```python
from build123d import *

# Parameters (mm, degrees)
CROQUIS1_W              = 800
CROQUIS1_H              = 342
SALIENTE_EXTRUIR1_DEPTH = 483
CROQUIS2_W              = 710
CROQUIS2_H              = 53.5
CORTAR_EXTRUIR1_DEPTH   = 483
CORTAR_EXTRUIR2_DEPTH   = 342
CORTAR_EXTRUIR4_DEPTH   = 800
VACIADO2_START          = -265.15812527
VACIADO2_OUTLINE_W      = 105
VACIADO2_OUTLINE_H      = 225
VACIADO2_DEPTH          = 530.31625054
VACIADO2_START_2        = -395
VACIADO2_2_DEPTH        = 790
VACIADO2_3_DEPTH        = 40
VACIADO2_START_3        = 355
VACIADO2_4_DEPTH        = 40
VACIADO2_START_4        = -112.5
VACIADO2_5_DEPTH        = 225
CROQUIS8_W              = 171
CROQUIS8_H              = 72.679369328
CORTAR_EXTRUIR7_DEPTH   = 113
CROQUIS9_W              = 171
CROQUIS9_H              = 72.679369328
CORTAR_EXTRUIR8_DEPTH   = 113


with BuildPart() as part:
    # Croquis1 → Saliente-Extruir1 (new body)
    with BuildSketch(Plane(origin=(0, 0, 0), x_dir=(1, 0, 0), z_dir=(0, 1, 0))):
        Rectangle(CROQUIS1_W, CROQUIS1_H)
    extrude(amount=SALIENTE_EXTRUIR1_DEPTH)

    # Croquis2 → Cortar-Extruir1 (cut)
    with BuildSketch(Plane(origin=(0, 483, 0), x_dir=(1, 0, 0), z_dir=(0, 1, 0))):
        with Locations((0, 144.25)):
            Rectangle(CROQUIS2_W, CROQUIS2_H)
        with Locations((0, -144.25)):
            Rectangle(CROQUIS2_W, CROQUIS2_H)
    extrude(amount=-CORTAR_EXTRUIR1_DEPTH, mode=Mode.SUBTRACT)

    # Croquis3 → Cortar-Extruir2 (cut)
    with BuildSketch(Plane.XY.offset(171)):
        Polygon((-355, 317.779645743), (-355, 0), (355, 0), (355, 317.779645743), (331.5, 317.779645743), (244, 422.779645743), (-244, 422.779645743), (-331.5, 317.779645743), align=None)
        Polygon((267.5, 483), (355, 378), (400, 378), (400, 483), align=None)
        Polygon((-400, 483), (-400, 378), (-355, 378), (-267.5, 483), align=None)
    extrude(amount=-CORTAR_EXTRUIR2_DEPTH, mode=Mode.SUBTRACT)

    # Croquis4 → Cortar-Extruir4 (cut)
    with BuildSketch(Plane(origin=(400, 0, 0), x_dir=(0, 0, -1), z_dir=(1, 0, 0))):
        Polygon((171, 378), (171, 70), (117.5, 378), align=None)
        Polygon((-171, 70), (-117.5, 378), (-171, 378), align=None)
        Polygon((-127.5, 45), (127.5, 45), (127.5, 75), (80, 325), (-80, 325), (-127.5, 75), align=None)
    extrude(amount=-CORTAR_EXTRUIR4_DEPTH, mode=Mode.SUBTRACT)

    # Vaciado2: read off the stored shape, not the designer's step
    # Vaciado2 outline → Vaciado2 (cut)
    with BuildSketch(Plane.YZ.offset(VACIADO2_START)):
        with Locations((425.5, 0)):
            Rectangle(VACIADO2_OUTLINE_W, VACIADO2_OUTLINE_H)
    extrude(amount=VACIADO2_DEPTH, mode=Mode.SUBTRACT)

    # Vaciado2 2 outline → Vaciado2 2 (cut)
    with BuildSketch(Plane.YZ.offset(VACIADO2_START_2)):
        Polygon((373, -112.5), (373, 112.5), (317.779645743, 112.5), (317.779645743, 81.371867309), (325, 80), (325, -80), (317.779645743, -81.371867309), (317.779645743, -112.5), align=None)
    extrude(amount=VACIADO2_2_DEPTH, mode=Mode.SUBTRACT)

    # Vaciado2 3 outline → Vaciado2 3 (cut)
    with BuildSketch(Plane.YZ.offset(VACIADO2_START_2)):
        Polygon((69.568973838, 166), (5, 166), (5, -166), (69.568973838, -166), (373, -113.293636689), (373, -112.5), (317.779645743, -112.5), (317.779645743, -81.371867309), (75, -127.5), (45, -127.5), (45, 127.5), (75, 127.5), (317.779645743, 81.371867309), (317.779645743, 112.5), (373, 112.5), (373, 113.293636689), align=None)
    extrude(amount=VACIADO2_3_DEPTH, mode=Mode.SUBTRACT)

    # Vaciado2 4 outline → Vaciado2 4 (cut)
    with BuildSketch(Plane.YZ.offset(VACIADO2_START_3)):
        Polygon((69.568973838, 166), (5, 166), (5, -166), (69.568973838, -166), (373, -113.293636689), (373, -112.5), (317.779645743, -112.5), (317.779645743, -81.371867309), (75, -127.5), (45, -127.5), (45, 127.5), (75, 127.5), (317.779645743, 81.371867309), (317.779645743, 112.5), (373, 112.5), (373, 113.293636689), align=None)
    extrude(amount=VACIADO2_4_DEPTH, mode=Mode.SUBTRACT)

    # Vaciado2 5 outline → Vaciado2 5 (cut)
    with BuildSketch(Plane.XY.offset(VACIADO2_START_4)):
        Polygon((352.65812527, 373), (265.15812527, 478), (265.15812527, 397.389895419), (285.483038119, 373), align=None)
        Polygon((-265.15812527, 478), (-352.65812527, 373), (-285.483038119, 373), (-265.15812527, 397.389895419), align=None)
    extrude(amount=VACIADO2_5_DEPTH, mode=Mode.SUBTRACT)

    # Croquis8 → Cortar-Extruir7 (cut)
    with BuildSketch(Plane(origin=(395.409836066, 329.508196721, 0), x_dir=(0, 0, -1), z_dir=(0.7682212795973777, 0.6401843996644778, 0))):
        with Locations((0, 131.461866471)):
            Rectangle(CROQUIS8_W, CROQUIS8_H)
    extrude(amount=-CORTAR_EXTRUIR7_DEPTH, mode=Mode.SUBTRACT)

    # Croquis9 → Cortar-Extruir8 (cut)
    with BuildSketch(Plane(origin=(-395.409836066, 329.508196721, 0), x_dir=(0, 0, 1), z_dir=(-0.7682212795973777, 0.6401843996644778, 0))):
        with Locations((0, 131.461866471)):
            Rectangle(CROQUIS9_W, CROQUIS9_H)
    extrude(amount=-CORTAR_EXTRUIR8_DEPTH, mode=Mode.SUBTRACT)


solid = part.part
```
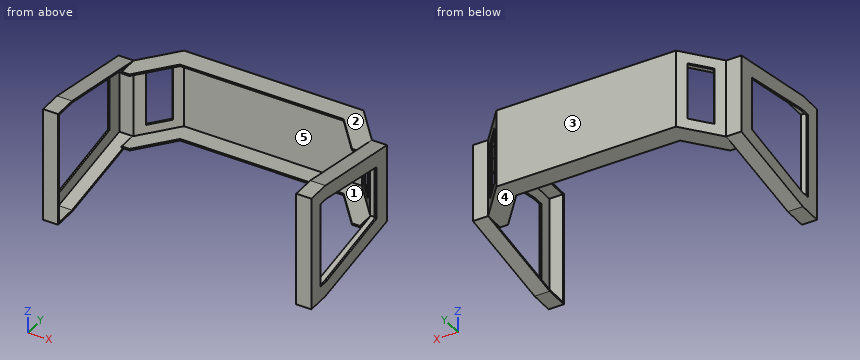
Here's how the part is built. I have some questions about the finished solid (model axes, mm). Face numbers are marked on the shaded views. A direction names the side the tool comes from. Coordinates: 2 decimals unless noted, no trailing zeros. Order: outer loops, then holes, each group sorted by start corner. A loop starts at its lowest first (then second) coordinate and runs counter-clockwise, first axis right, second up. Notation, with made-up numbers: M -30.75,-35.75 L 28.25,-35.75 A24 ccw 28.25,2.25 Z; hole C 63.25,73 d1. An arc over 180 degrees is marked long. Answer as a JSON object with one key per item and string values. Group by question number.
(1) Suppose I cut it at B-B, the plane z = 137.5. Please give me the cut outline in (x, y), then the cut area to 3 significant figures.
(2) Suppose I cut it at C-C, the plane y = 413. Please give me the cut outline in (x, z).
(3) Which directions (+Z, -Z, +X, -X, +Y, -Y) give clear straight access to the entire face, cutting with the end or side of a thin tool? Please do the marked faces 1 and 2.
(4) Suppose I cut it at D-D, the plane z = -56.5. State how many separate pieces and enclosed holes the cut face has, then the cut area to 4 significant figures.
(5) If we mould it in two halves opening along X, with no side actions, what happens to the marked faces 3, 4 and 5? For each: released by +X, released by -X, zero draft, split by the parting line, or undercut.
(6) I need wall thicknesses on probe 1 along X at (y, z) = (331.5, -88); probe 2 along Y at (x, z) = (-356.5, 14.5); probe 3 along Y at (x, z) = (-63.5, 75). Which ranges of each line are inside material? Lowest first, please.
(7) For pin 1 (4 mm diameter, centred on x = -343, z = -114, fed in from -Y); pin 2 (3 mm diameter, centred on y = 396.5, z = 110, fed in from +X); pin 3 (2.5 mm diameter, centred on x = -35.5, z = 115, fed in from -Y); pin 4 (6 mm diameter, centred on y = 398.5, z = 121, fed in from +X), each with a flat end and sliding along its axis, tell me the tip position at first contact or that it passes through.
(8) Suppose I cut it at A-A, the plane x = -122. Please give me the cut outline in (y, z), then the cut area to 3 significant figures.
Values found:
{
 "1": {"outline": "M -400,0 L -355,0 L -355,5 L -395,5 L -395,233.64 L -355,233.64 L -355,262.86 L -400,262.86 Z; M 355,0 L 400,0 L 400,262.86 L 355,262.86 L 355,233.64 L 395,233.64 L 395,5 L 355,5 Z", "area": "5,370 mm^2"},
 "2": {"outline": "M -325.83,-117.5 L -252.15,-117.5 L -252.15,-112.5 L -319.32,-112.5 L -319.32,-85.5 L -325.83,-85.5 Z; M -325.83,85.5 L -319.32,85.5 L -319.32,112.5 L -252.15,112.5 L -252.15,117.5 L -325.83,117.5 Z; M 252.15,-117.5 L 325.83,-117.5 L 325.83,-85.5 L 319.32,-85.5 L 319.32,-112.5 L 252.15,-112.5 Z; M 252.15,112.5 L 319.32,112.5 L 319.32,85.5 L 325.83,85.5 L 325.83,117.5 L 252.15,117.5 Z"},
 "3": {"face 1": "-Y", "face 2": "+Z, +Y, -Y"},
 "4": {"separate pieces": "5", "enclosed holes": "0", "area": "5,095 mm^2"},
 "5": {"face 3": "zero draft", "face 4": "undercut", "face 5": "undercut"},
 "6": {"probe 1": "x = -400 to -395, 395 to 400", "probe 2": "y = 0 to 5, 373 to 378", "probe 3": "y = 478 to 483"},
 "7": {"pin 1": "stops at y = 317.78", "pin 2": "stops at x = 340.83", "pin 3": "stops at y = 422.78", "pin 4": "passes through"},
 "8": {"outline": "M 422.78,-117.5 L 483,-117.5 L 483,117.5 L 422.78,117.5 L 422.78,112.5 L 478,112.5 L 478,-112.5 L 422.78,-112.5 Z", "area": "1,730 mm^2"}
}
